The listing builds one solid part. Answer for the finished solid, in the listing's coordinates (mm). Face numbers are marked on the shaded views. A direction names the side the tool comes from. Coordinates: 2 decimals unless noted, no trailing zeros. Loops run counter-clockwise (first coordinate to the right, second up) from the corner with the lowest first, then second, coordinate; pieces in that order, holes last. Notation, with made-up numbers: (15.5, 37) - (29.5, 37) arc R29 ccw to (29.5, 66) - close; hole circle Ø4 at (-30.75, 49). An arc over 180 degrees is marked (long way). Return JSON: item names as keys, results as strings. Group by question number.
1. Section B-B (z = 14.75) is taken. Write down the section's boundary in (x, y), and give its area (3 significant figures).
2. Each of these flat-tipped pins is pushed along its axis until it touches: P1, Ø4, axis at y = -1.5, z = 16.5, coming from the -X side; P2, Ø3, axis at x = -12.5, y = 2, coming from the -Z side; P3, Ø3.5, axis at x = 0, z = 21.5, coming from the +Y side. Where does it stop, or does it pass through?
3. The mould has two halves that part along X. Classify the marked faces 6, 7 and 8: pulls with the +X half, pulls with the -X half, needs draft (parallel to the pull), parting line crosses it, or undercut.
4. Find the intervals of material crossed by line 1 along Y through (x, z) = (12.5, 26.15); line 2 along X through (y, z) = (2.25, 21.25); line 3 along Y through (x, z) = (12.5, 22), in increasing order.
5. Section C-C (z = 26.75) is taken. Write down the section's boundary in (x, y).
6. Which of the six approach directions +Z, -Z, +X, -X, +Y, -Y give full straight-line access (tool end or side, diameter ignored) to the marked faces 1, 2, 3, 4 and 5?
7. Section D-D (y = -3.25) is taken. Write down the section's boundary in (x, z), and give its area (3 significant figures).
8. Section A-A (x = 0) is taken. Write down the section's boundary in (y, z).
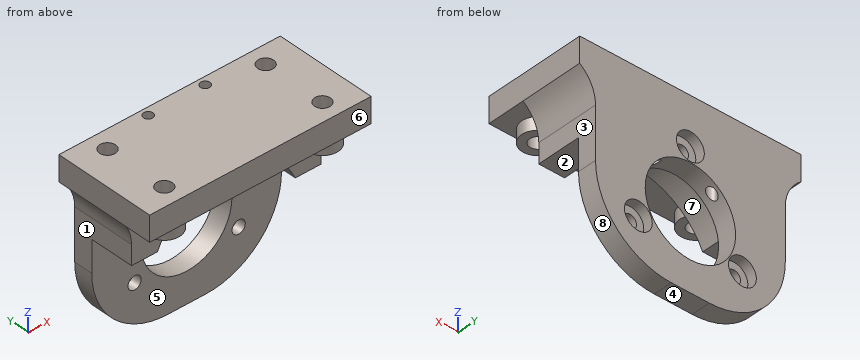
```python
from build123d import *

# Parameters (mm, degrees)
SKETCH1_W                           = 30
SKETCH1_H                           = 10
MAIN_DEPTH                          = 25
SKETCH5_R                           = 1.05
SKETCH5_R_2                         = 7.15
MAINANDFIXHOLE_DEPTH                = 31.822070015
SKETCH6_R                           = 2.2
CODERFIXHOLE2_DEPTH                 = 1.5
CODERHOLE2_DEPTH                    = 7
SKETCH10_W                          = 35
SKETCH10_H                          = 16
LINK_DEPTH                          = 4
SKETCH8_R                           = 1.25
VERTICALHOLES_DEPTH                 = 12
SKETCH13_R                          = 2.5
LINKREINFORCEMENT_DEPTH             = 2
FILLET4_R                           = 6
FILLET6_R                           = 12
HOLELPATTERN1_COUNT                 = 2
HOLELPATTERN1_PITCH                 = 25
HOLELPATTERN1_COUNT_DIR2            = 2
HOLELPATTERN1_PITCH_DIR2            = 10
HOLETOACCESSENCODERSCREW_REACH      = 37.612
HOLETOACCESSENCODERSCREW_END_RADIUS = 7.15
SKETCH14_R                          = 0.75


with BuildPart() as part:
    # Sketch1 → Main (new body)
    with BuildSketch(Plane.XY):
        Rectangle(SKETCH1_W, SKETCH1_H)
    extrude(amount=MAIN_DEPTH)

    # Sketch5 → MainAndFixHole (cut, through all)
    with BuildSketch(Plane(origin=(0, -5, 0), x_dir=(-1, 0, 0), z_dir=(0, -1, 0))):
        with Locations(Location((0, -21.5, 0), (0, 0, 90))):
            Circle(SKETCH5_R)
        with Locations(Location((-8.227241336, -7.25, 0), (0, 0, 90))):
            Circle(SKETCH5_R)
        with Locations(Location((8.227241336, -7.25, 0), (0, 0, 90))):
            Circle(SKETCH5_R)
        with Locations(Location((0, -12, 0), (0, 0, 90))):
            Circle(SKETCH5_R_2)
    extrude(amount=-MAINANDFIXHOLE_DEPTH, mode=Mode.SUBTRACT)

    # Sketch6 → CoderFixHole2 (cut)
    with BuildSketch(Plane(origin=(0, 5, 0), x_dir=(-1, 0, 0), z_dir=(0, -1, 0))):
        with Locations(Location((0, -21.5, 0), (0, 0, 90))):
            Circle(SKETCH6_R)
        with Locations(Location((-8.227241336, -7.25, 0), (0, 0, 90))):
            Circle(SKETCH6_R)
        with Locations(Location((8.227241336, -7.25, 0), (0, 0, 90))):
            Circle(SKETCH6_R)
    extrude(amount=CODERFIXHOLE2_DEPTH, mode=Mode.SUBTRACT)

    # Sketch11 → CoderHole2 (cut)
    with BuildSketch(Plane(origin=(0, -5, 0), x_dir=(1, 0, 0), z_dir=(0, 1, 0))):
        with BuildLine():
            Line((-15, 0), (15, 0))
            Line((15, 0), (15, -17))
            Line((15, -17), (10.908712115, -17))
            ThreePointArc((10.908712115, -17), (0, -24), (-10.908712115, -17))
            Line((-10.908712115, -17), (-15, -17))
            Line((-15, -17), (-15, 0))
        make_face()
    extrude(amount=CODERHOLE2_DEPTH, mode=Mode.SUBTRACT)

    # Sketch10 → Link (add)
    with BuildSketch(Plane.XY.offset(25)):
        with Locations((0, -3)):
            Rectangle(SKETCH10_W, SKETCH10_H)
    extrude(amount=LINK_DEPTH)

    # Sketch8 → VerticalHoles (cut)
    with BuildSketch(Plane.XY.offset(29)):
        with Locations((12.5, 2)):
            Circle(SKETCH8_R)
    verticalholes = extrude(amount=-VERTICALHOLES_DEPTH, mode=Mode.SUBTRACT)

    # Sketch13 → LinkReinforcement (add)
    with BuildSketch(Plane(origin=(0, 0, 25), x_dir=(-1, 0, 0), z_dir=(0, 0, -1))):
        with Locations((-12.5, -8)):
            Circle(SKETCH13_R)
        with Locations((12.5, -8)):
            Circle(SKETCH13_R)
    extrude(amount=LINKREINFORCEMENT_DEPTH)

    # Fillet4
    # the kernel refuses this fillet: 6 mm, written as the material it adds along each edge
    with BuildSketch(Plane(origin=(15, -5, 25), x_dir=(1, 0, 0), z_dir=(0, 1, 0)), Plane(origin=(-15, 5, 25), x_dir=(-1, 0, 0), z_dir=(0, -1, 0))) as fillet4_piece_1:
        with BuildLine():
            CenterArc((6, 4.873397172), FILLET4_R, 180, 54.314665287)
            Line((0, 4.873397172), (-0.12, 4.873397172))
            Line((-0.12, 4.873397172), (-0.12, 0))
            Line((-0.12, 0), (0, -0.12))
            ThreePointArc((0, -0.12), (1.25, -0.12), (2.43, -0.097467943))
            Line((2.43, -0.097467943), (2.5, 0))
        make_face()
    extrude(amount=10)

    # Fillet6
    fillet6_edges = [part.edges().sort_by_distance(p)[0] for p in [
        (-15, 3.5, 0),
        (15, 3.5, 0),
    ]]
    fillet(fillet6_edges, radius=FILLET6_R)

    # HoleLPattern1: VerticalHoles 2 × 2
    with Locations(*[(-i * HOLELPATTERN1_PITCH, -j * HOLELPATTERN1_PITCH_DIR2, 0) for i in range(HOLELPATTERN1_COUNT) for j in range(HOLELPATTERN1_COUNT_DIR2) if (i, j) != (0, 0)]):
        add(verticalholes, mode=Mode.SUBTRACT)

    # HoleToAccessEncoderScrew: up to this cylinder (the profile starts outside it)
    holetoaccessencoderscrew_end = Plane(origin=(0, 3.75, 12), z_dir=(0, -1, 0)) * Cylinder(HOLETOACCESSENCODERSCREW_END_RADIUS, 90.524, mode=Mode.PRIVATE)
    # Sketch14 → HoleToAccessEncoderScrew (cut, up to the surface)
    with BuildSketch(Plane.XY.offset(29), mode=Mode.PRIVATE) as holetoaccessencoderscrew_sk1:
        with Locations((4.5, 3.75)):
            Circle(SKETCH14_R)
    holetoaccessencoderscrew_tool1 = extrude(holetoaccessencoderscrew_sk1.sketch, amount=-HOLETOACCESSENCODERSCREW_REACH, mode=Mode.PRIVATE) - holetoaccessencoderscrew_end
    add(holetoaccessencoderscrew_tool1.solids().sort_by_distance((4.5, 3.75, 29))[0], mode=Mode.SUBTRACT)
    # Sketch14 → HoleToAccessEncoderScrew (cut, up to the surface)
    with BuildSketch(Plane.XY.offset(29), mode=Mode.PRIVATE) as holetoaccessencoderscrew_sk2:
        with Locations((-4.5, 3.75)):
            Circle(SKETCH14_R)
    holetoaccessencoderscrew_tool2 = extrude(holetoaccessencoderscrew_sk2.sketch, amount=-HOLETOACCESSENCODERSCREW_REACH, mode=Mode.PRIVATE) - holetoaccessencoderscrew_end
    add(holetoaccessencoderscrew_tool2.solids().sort_by_distance((-4.5, 3.75, 29))[0], mode=Mode.SUBTRACT)


solid = part.part
```
The answers:
{
 "1": {"outline": "(-15, 2) - (-6.6, 2) - (-6.6, 5) - (-15, 5) - close; (6.6, 2) - (15, 2) - (15, 5) - (6.6, 5) - close", "area": "50.4 mm2"},
 "2": {"P1": "stops at x = -15", "P2": "stops at z = 3.06", "P3": "stops at y = 3.5"},
 "3": {"face 6": "needs draft", "face 7": "undercut", "face 8": "pulls with the +X half"},
 "4": {"line 1": "y = -11 to -9.25, -6.75 to 0.75, 3.25 to 5", "line 2": "x = -15.11 to -13.72, -11.28 to -1.02, 1.02 to 11.28, 13.72 to 15.11", "line 3": "y = -5 to 0.75, 3.25 to 5"},
 "5": {"outline": "(-17.5, -11) - (17.5, -11) - (17.5, 5) - (-17.5, 5) - close; hole circle Ø2.5 at (-12.5, -8); hole circle Ø2.5 at (-12.5, 2); hole circle Ø1.5 at (-4.5, 3.75); hole circle Ø1.5 at (4.5, 3.75); hole circle Ø2.5 at (12.5, -8); hole circle Ø2.5 at (12.5, 2)"},
 "6": {"face 1": "-Z, -X, +Y, -Y", "face 2": "-Z, +X, -X, -Y", "face 3": "-Z, +X, +Y, -Y", "face 4": "-Z, +X, -X, +Y, -Y", "face 5": "-Z, -Y"},
 "7": {"outline": "(-17.5, 25) arc R6 cw to (-15, 20.13) - (-15, 17) - (-10.91, 17) arc R12 cw to (10.91, 17) - (15, 17) - (15, 20.13) arc R6 cw to (17.5, 25) - (17.5, 29) - (-17.5, 29) - close", "area": "278 mm2"},
 "8": {"outline": "(-11, 25) - (-5, 25) - (-5, 24) - (2, 24) - (2, 22.55) - (3.5, 22.55) - (3.5, 23.7) - (5, 23.7) - (5, 29) - (-11, 29) - close; (2, 0) - (5, 0) - (5, 4.85) - (2, 4.85) - close; (2, 19.15) - (5, 19.15) - (5, 19.3) - (3.5, 19.3) - (3.5, 20.45) - (2, 20.45) - close"}
}
